The model under review builds one solid part; all positions refer to its coordinate system, in mm. A direction names the side the tool comes from. Coordinates: 2 decimals unless noted, no trailing zeros. Loops run counter-clockwise (first coordinate to the right, second up) from the corner with the lowest first, then second, coordinate; pieces in that order, holes last. Notation, with made-up numbers: (17.5, 21) - (22.5, 21) arc R38 cw to (22.5, 59) - close; hole circle Ø7 at (86.5, -21.75). An arc over 180 degrees is marked (long way). One line per item, written item: value. Start each with the question number.
1. For faces 1 (the face through (-13.57, 0.45, 0.14)), 2 (the face through (-0.126, 19.715, -9.699)), list the 3-axis set-ups (+Z, -Z, +X, -X, +Y, -Y) from which the entire face can be reached by the end or side of a thin tool; tool diameter is ignored.
2. Mouldability with a two-part tool opening along Z and no side actions: class faces 3 (the face through (10.43, 0.45, 0.16)), 4 (the face through (-9.699, 10.372, -9.715)), 5 (the face through (0, 24, 0)), 6 (the face through (-12.797, 10.62, 12.859)) as +Z half, -Z half, draft (parallel to the pull), parting line (faces both ways), or undercut.
3. We need section C-C, the plane z = 1.25. Give the boundary of the cut face in (x, y), then the cut area to 3 significant figures.
4. We need section B-B, the plane x = -4.25. Give the boundary of the cut face in (y, z), then the cut area to 3 significant figures.
5. Insertion check: P1, Ø5, axis at x = -7, z = 5.5, coming from the -Y side; P2, Ø1, axis at x = 5.5, z = -10, coming from the -Y side; P3, Ø5.5, axis at x = -2, z = -2, coming from the -Y side. Each pin has a flat end and moves straight along its axis. Give the tip position at first contact, or say it passes through.
6. To check wall thickness, follow line 1 (X direction, y = 6, z = -7.5); line 2 (Y direction, x = 9, z = -2.5). State the ranges of each line that lie inside material, in increasing order.
7. We need section A-A, the plane y = 8.5. Give the boundary of the cut face in (x, z), then the cut area to 3 significant figures.
8. We need section D-D, the plane y = 21. Give the boundary of the cut face in (x, z), then the cut area to 3 significant figures.
Autodesk Inventor part; units mm, degrees
ref_plane "YZ Plane" through (0, 0, 0) normal (1, 0, 0) x (0, 1, 0)
ref_plane "XZ Plane" through (0, 0, 0) normal (0, 1, 0) x (-1, 0, 0)
ref_plane "XY Plane" through (0, 0, 0) normal (0, 0, 1) x (1, 0, 0)
sketch "Sketch1" plane through (0, 0, 0) normal (0, 1, 0) x (-1, 0, 0)
  line L0 (-10, 10) -> (10, 10)
  line L1 (10, 10) -> (10, -10)
  line L2 (10, -10) -> (-10, -10)
  line L3 (-10, -10) -> (-10, 10)
  line L4 (-10, 10) -> (10, -10) construction
  line L5 (10, 10) -> (-10, -10) construction
  line L6 (14, -10) -> (14, 10)
  line L7 (10, 14) -> (-10, 14)
  line L8 (-14, 10) -> (-14, -10)
  line L9 (-10, -14) -> (10, -14)
  arc A0 (10, -14) -> (14, -10) centre (10, -10) ccw
  arc A1 (-14, -10) -> (-10, -14) centre (-10, -10) ccw
  arc A2 (-10, 14) -> (-14, 10) centre (-10, 10) ccw
  arc A3 (14, 10) -> (10, 14) centre (10, 10) ccw
  point P0 (0, 0)
  point P1 (14, -14)
  point P2 (14, 14)
  point P3 (-14, 14)
  point P4 (-14, -14)
  dimension "d0" = 20
  dimension "d1" = 4
  dimension "d6" = 4
extrude "Extrusion1" add sketch "Sketch1" along normal blind 20
sketch "Sketch2" plane through (0, 20, 0) normal (0, 1, 0) x (1, 0, 0)
  line L0 (-10, -14) -> (10, -14)
  line L1 (-14, 10) -> (-14, -10)
  line L2 (10, 14) -> (-10, 14)
  line L3 (14, -10) -> (14, 10)
  arc A0 (-10, 14) -> (-14, 10) centre (-10, 10) ccw
  arc A1 (-14, -10) -> (-10, -14) centre (-10, -10) ccw
  arc A2 (10, -14) -> (14, -10) centre (10, -10) ccw
  arc A3 (14, 10) -> (10, 14) centre (10, 10) ccw
  point P0 (0, 0)
  point P1 (-13, -13)
  point P2 (13, -13)
  point P3 (-13, 13)
  point P4 (13, 13)
extrude "Extrusion2" add sketch "Sketch2" along normal blind 4
fillet "Fillet1" radius 4 8 edges at (12.8284, 24, 12.8284) (14, 24, 0) (12.8284, 24, -12.8284) (0, 24, -14) (-12.8284, 24, -12.8284) (-14, 24, 0) (-12.8284, 24, 12.8284) (0, 24, 14)
fillet "Fillet2" radius 1.5 12 edges at (12.8284, 0, 12.8284) (14, 0, 0) (12.8284, 0, -12.8284) (0, 0, -14) (-12.8284, 0, -12.8284) (-14, 0, 0) (-12.8284, 0, 12.8284) (0, 0, 14) (0, 0, 10) (10, 0, 0) (0, 0, -10) (-10, 0, 0)
fillet "Fillet3" radius 1 8 edges at (10, 10.75, 10) (10.4393, 0.4393, 10.4393) (10, 10.75, -10) (10.4393, 0.4393, -10.4393) (-10, 10.75, -10) (-10.4393, 0.4393, -10.4393) (-10, 10.75, 10) (-10.4393, 0.4393, 10.4393)
fillet "Fillet4" radius 1 8 edges at (9.7071, 20, 9.7071) (0, 20, 10) (-9.7071, 20, 9.7071) (-10, 20, 0) (-9.7071, 20, -9.7071) (0, 20, -10) (9.7071, 20, -9.7071) (10, 20, 0)
properties part number "Cap_3DPrint"
Findings below:
1. face 1: +Z, -Z, -X, -Y
1. face 2: -Y
2. face 3: undercut
2. face 4: undercut
2. face 5: draft
2. face 6: +Z half
3. outline: (-14, 1.5) arc R1.5 ccw to (-12.5, 0) - (-11.5, 0) arc R1.5 ccw to (-10, 1.5) - (-10, 19) arc R1 cw to (-9, 20) - (9, 20) arc R1 cw to (10, 19) - (10, 1.5) arc R1.5 ccw to (11.5, 0) - (12.5, 0) arc R1.5 ccw to (14, 1.5) - (14, 20) arc R4 ccw to (10, 24) - (-10, 24) arc R4 ccw to (-14, 20) - close
3. area: 264 mm2
4. outline: (0, -12.5) arc R1.5 ccw to (1.5, -14) - (20, -14) arc R4 ccw to (24, -10) - (24, 10) arc R4 ccw to (20, 14) - (1.5, 14) arc R1.5 ccw to (0, 12.5) - (0, 11.5) arc R1.5 ccw to (1.5, 10) - (19, 10) arc R1 cw to (20, 9) - (20, -9) arc R1 cw to (19, -10) - (1.5, -10) arc R1.5 ccw to (0, -11.5) - close
4. area: 264 mm2
5. P1: y = 19.87
5. P2: y = 0.38
5. P3: y = 20
6. line 1: -14 to -10, 10 to 14
6. line 2: 20 to 24
7. outline: (-14, -10) arc R4 ccw to (-10, -14) - (10, -14) arc R4 ccw to (14, -10) - (14, 10) arc R4 ccw to (10, 14) - (-10, 14) arc R4 ccw to (-14, 10) - close; hole (-10, -9) arc R1 ccw to (-9, -10) - (9, -10) arc R1 ccw to (10, -9) - (10, 9) arc R1 ccw to (9, 10) - (-9, 10) arc R1 ccw to (-10, 9) - close
7. area: 371 mm2
8. outline: (-13.87, -10) arc R3.87 ccw to (-10, -13.87) - (10, -13.87) arc R3.87 ccw to (13.87, -10) - (13.87, 10) arc R3.87 ccw to (10, 13.87) - (-10, 13.87) arc R3.87 ccw to (-13.87, 10) - close
8. area: 757 mm2
